Verification items for the finished model (mm, model axes). Face numbers are marked on the shaded views. A direction names the side the tool comes from. Give positions to 0.01 mm unless a question says otherwise; leave off trailing zeros. Order: outer loops, then holes, each group sorted by start corner. A loop starts at its lowest first (then second) coordinate and runs counter-clockwise, first axis right, second up. Notation, with made-up numbers: M 4,89 L 46,89 A24 ccw 46,105 Z; hole C -3.75,-34.75 d7. An arc over 180 degrees is marked long. Answer as a JSON object with one key per item and string values.
```python
from build123d import *

# Parameters (mm, degrees)
ESQUISSE1_R             = 7.7
BOSS_EXTRU_1_DEPTH      = 2.8
ESQUISSE2_R             = 1.9
BOSS_EXTRU_2_DEPTH      = 30
ESQUISSE3_R             = 1.65
ENL_V_MAT_EXTRU_1_DEPTH = 32.91520014
CONG_2_R                = 1
ESQUISSE4_R             = 2.1
ESQUISSE4_R_2           = 1.9
BOSS_EXTRU_3_DEPTH      = 3
CONG_3_R                = 1
CONG_4_R                = 2
ESQUISSE5_W             = 0.7
ESQUISSE5_H             = 1.4
ENL_V_MAT_EXTRU_2_DEPTH = 30.113227234


# Some blends are built 0.0001 mm under size
with BuildPart() as part:
    # Esquisse1 → Boss.-Extru.1 (new body)
    with BuildSketch(Plane.XY):
        Circle(ESQUISSE1_R)
    extrude(amount=BOSS_EXTRU_1_DEPTH)

    # Esquisse2 → Boss.-Extru.2 (add)
    with BuildSketch(Plane.XY.offset(2.8)):
        with Locations((0, 4.8)):
            Circle(ESQUISSE2_R)
    extrude(amount=BOSS_EXTRU_2_DEPTH)

    # Esquisse3 → Enlèv. mat.-Extru.1 (cut, through all)
    with BuildSketch(Plane.XY.offset(2.8)):
        Circle(ESQUISSE3_R)
    extrude(amount=-ENL_V_MAT_EXTRU_1_DEPTH, mode=Mode.SUBTRACT)

    # Congé2
    cong_2_edges = [part.edges().sort_by_distance(p)[0] for p in [
        (-1.9, 4.8, 2.8),
    ]]
    fillet(cong_2_edges, radius=CONG_2_R - 0.0001)  # a hair under: the kernel refuses the full size

    # Esquisse4 → Boss.-Extru.3 (add)
    with BuildSketch(Plane.XY.offset(5.8)):
        with Locations((0, 4.8)):
            Circle(ESQUISSE4_R)
        with Locations((0, 4.8)):
            Circle(ESQUISSE4_R_2, mode=Mode.SUBTRACT)
    extrude(amount=BOSS_EXTRU_3_DEPTH)

    # Congé3
    # the kernel refuses this fillet: 1 mm, written as the material it adds along each edge
    with BuildSketch(Plane(origin=(0, 4.8, 5.8), x_dir=(1, 0, 0), z_dir=(0, -1, 0))) as cong_3_piece_1:
        with BuildLine():
            CenterArc((2.9, -0.6), CONG_3_R, 143.130102354, 36.869897646)
            Line((2.1, 0), (2.084, 0.012))
            ThreePointArc((2.084, 0.012), (2, 0.02), (1.9, 0.02))
            Line((1.9, 0.02), (1.88, 0))
            Line((1.88, 0), (1.88, -0.6))
            Line((1.88, -0.6), (1.9, -0.6))
        make_face()
    revolve(axis=Axis((0, 4.8, 5.8), (0, 0, 1)))
    with BuildSketch(Plane(origin=(0, 4.8, 8.8), x_dir=(1, 0, 0), z_dir=(0, -1, 0))) as cong_3_piece_2:
        with BuildLine():
            CenterArc((2.9, 0.6), CONG_3_R, 180, 36.869897646)
            Line((1.9, 0.6), (1.88, 0.6))
            Line((1.88, 0.6), (1.88, 0))
            Line((1.88, 0), (1.9, -0.02))
            ThreePointArc((1.9, -0.02), (2, -0.02), (2.084, -0.012))
            Line((2.084, -0.012), (2.1, 0))
        make_face()
    revolve(axis=Axis((0, 4.8, 8.8), (0, 0, 1)))

    # Congé4
    cong_4_edges = [part.edges().sort_by_distance(p)[0] for p in [
        (-2.1, 4.8, 8.8),
        (-2.1, 4.8, 5.8),
    ]]
    fillet(cong_4_edges, radius=CONG_4_R)

    # Esquisse5 → Enlèv. mat.-Extru.2 (cut, through all)
    with BuildSketch(Plane.XY.offset(5.8)):
        with Locations((0, 6.7)):
            Rectangle(ESQUISSE5_W, ESQUISSE5_H)
    extrude(amount=ENL_V_MAT_EXTRU_2_DEPTH, mode=Mode.SUBTRACT)


solid = part.part
```
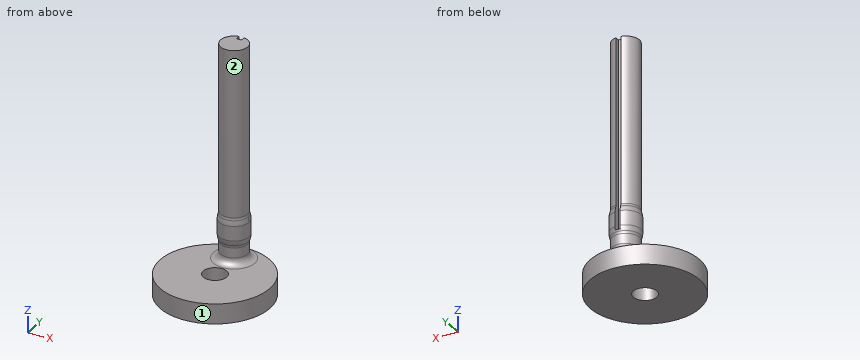
Q1. Material ranges on L1, parallel to Y at x = 0, z = 1.85; L2, parallel to Z at x = 2, y = -5.5; L3, parallel to Y at x = -4.25, z = 2.5, recorded low to high.
Resolved:
{"L1": "y = -7.7 to -1.65, 1.65 to 7.7", "L2": "z = 0 to 2.8", "L3": "y = -6.42 to 6.42"}
Q2. Gauge pin test, flat ends, axial feed: pin 1 Ø2 at (x, z) = (-1, 8.5) entering from -Y; pin 2 Ø3 at (x, y) = (0, 0) entering from -Z; pin 3 Ø5 at (y, z) = (4.5, 9.5) entering from -X; pin 4 Ø2 at (x, y) = (-1.5, -4.5) entering from +Z. Record the tip position at first contact, or that the pin passes through.
Resolved:
{"pin 1": "stops at y = 2.7", "pin 2": "passes through", "pin 3": "stops at x = -2.1", "pin 4": "stops at z = 2.8"}
Q3. Section check B-B on z = 4.5. Record the cut outline in (x, y).
Resolved:
{"outline": "C 0,4.8 d3.8"}
Q4. Section check C-C on x = 6.5. Record the cut outline in (y, z).
Resolved:
{"outline": "M -4.13,0 L 4.13,0 L 4.13,2.8 L -4.13,2.8 Z"}
Q5. Tool access check on the marked faces 1 and 2. Record the directions out of +Z, -Z, +X, -X, +Y, -Y that give a thin tool (end or side, any length) a straight path to the whole face; none if there is none.
Resolved:
{"face 1": "+Z, -Z", "face 2": "+Z"}
Q6. Section check A-A on y = 0. Record the cut outline in (x, z).
Resolved:
{"outline": "M -7.7,0 L -1.65,0 L -1.65,2.8 L -7.7,2.8 Z; M 1.65,0 L 7.7,0 L 7.7,2.8 L 1.65,2.8 Z"}
Q7. Section check D-D on y = -3. Record the cut outline in (x, z).
Resolved:
{"outline": "M -7.09,0 L 7.09,0 L 7.09,2.8 L -7.09,2.8 Z"}
